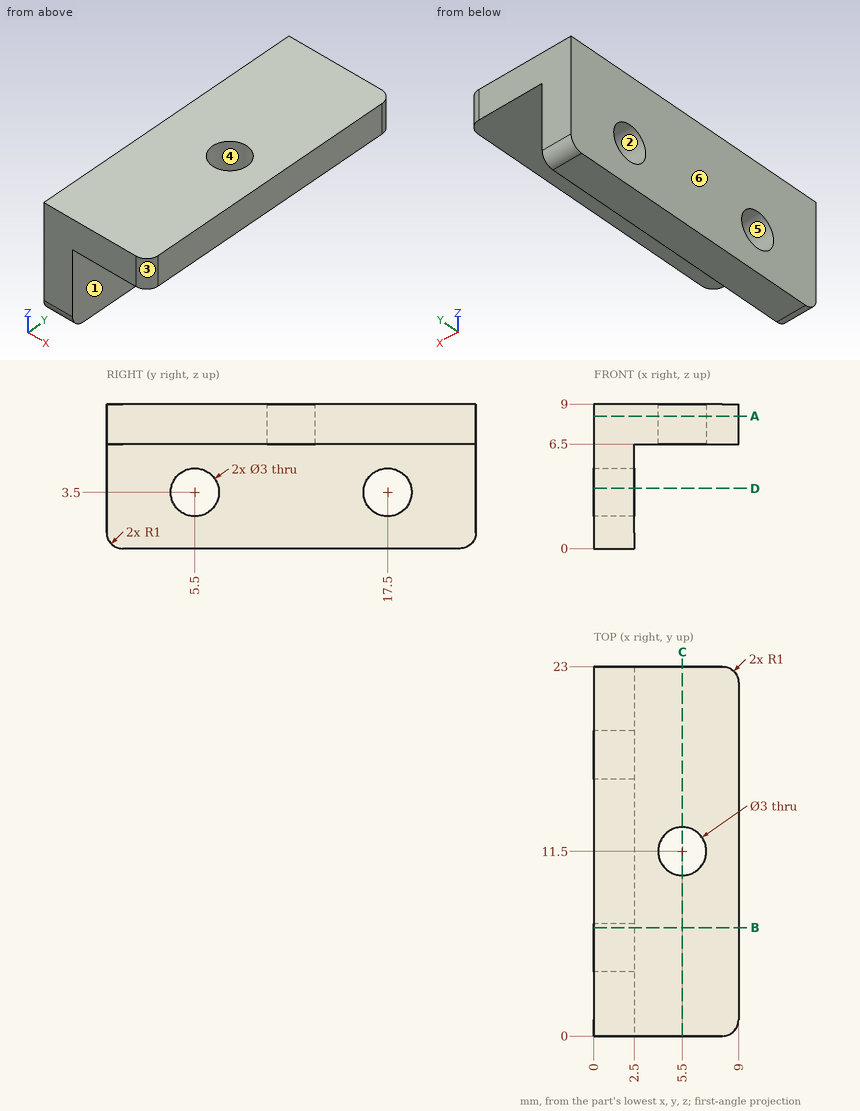
Design review of the part shown in the three views and the two pictorial views. Dimensions are in mm from the part's minimum x, y and z. A direction names the side the tool comes from. Coordinates: 2 decimals unless noted, no trailing zeros. Order: outer loops, then holes, each group sorted by start corner. A loop starts at its lowest first (then second) coordinate and runs counter-clockwise, first axis right, second up.
1) Wall thickness on line 1 along Y through (x, z) = (1.75, 3.5); line 2 along Y through (x, z) = (1, 3); line 3 along Z through (x, y) = (7.25, 14): over which ranges is each line inside the solid? List them lowest first.
2) Take a section at C-C, the plane x = 5.5. Give the boundary of the cut face in (y, z), and give its area (3 significant figures).
3) Take a section at B-B, the plane y = 6.75. Give the boundary of the cut face in (x, z).
4) For the marked faces 1 and 2, list the 3-axis set-ups (+Z, -Z, +X, -X, +Y, -Y) from which the entire face can be reached by the end or side of a thin tool; tool diameter is ignored.
5) Take a section at A-A, the plane z = 8.25. Give the boundary of the cut face in (x, y), and give its area (3 significant figures).
6) Clearance check with flat-ended pins moving along their axes: pin 1 (2.5 mm diameter, centred on y = 5.5, z = 3.5, fed in from +X); pin 2 (5 mm diameter, centred on y = 12.5, z = 3, fed in from +X); pin 3 (3.5 mm diameter, centred on x = 5.5, y = 11.5, fed in from -Z). State where each tip first meets the part, or that it passes through.
7) Mouldability with a two-part tool opening along X and no side actions: class the marked faces 3, 4, 5 and 6 as +X half, -X half, draft (parallel to the pull), parting line (faces both ways), or undercut.
8) Take a section at D-D, the plane z = 3.75. Give the boundary of the cut face in (x, y).
Returned:
1. line 1: y = 0 to 4, 7 to 16, 19 to 23
1. line 2: y = 0 to 4.09, 6.91 to 16.09, 18.91 to 23
1. line 3: z = 6.5 to 9
2. outline: (0, 6.5) - (10, 6.5) - (10, 9) - (0, 9) - close; (13, 6.5) - (23, 6.5) - (23, 9) - (13, 9) - close
2. area: 50.0 mm2
3. outline: (0, 0) - (2.5, 0) - (2.5, 2.67) - (0, 2.67) - close; (0, 4.33) - (2.5, 4.33) - (2.5, 6.5) - (9, 6.5) - (9, 9) - (0, 9) - close
4. face 1: -Z, +X, +Y, -Y
4. face 2: +X, -X
5. outline: (0, 0) - (8, 0) arc R1 ccw to (9, 1) - (9, 22) arc R1 ccw to (8, 23) - (0, 23) - close; hole circle Ø3 at (5.5, 11.5)
5. area: 200 mm2
6. pin 1: passes through
6. pin 2: stops at x = 2.5
6. pin 3: stops at z = 6.5
7. face 3: +X half
7. face 4: undercut
7. face 5: draft
7. face 6: -X half
8. outline: (0, 0) - (2.5, 0) - (2.5, 4.02) - (0, 4.02) - close; (0, 6.98) - (2.5, 6.98) - (2.5, 16.02) - (0, 16.02) - close; (0, 18.98) - (2.5, 18.98) - (2.5, 23) - (0, 23) - close
